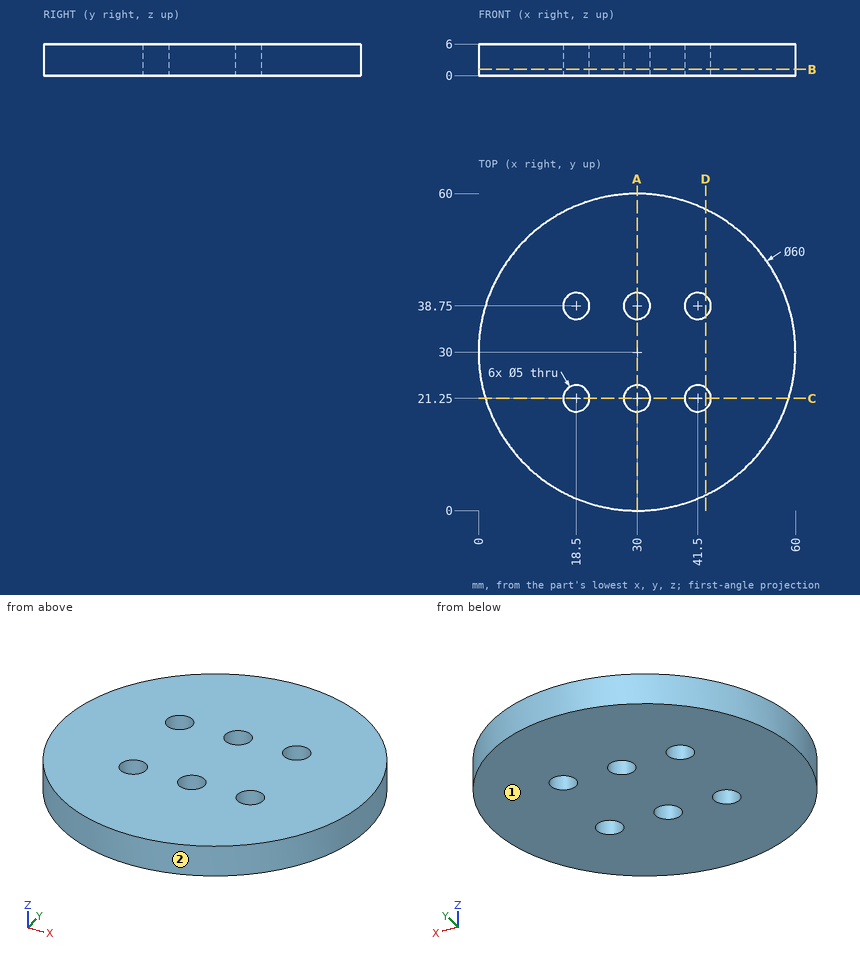
Answer from the drawing. Dimensions are ordinates in mm from the lowest x, y and z of the part. Coordinates: 2 decimals unless noted, no trailing zeros. Loops run counter-clockwise (first coordinate to the right, second up) from the corner with the lowest first, then second, coordinate; pieces in that order, holes last.
Q1. The part is cut by section B-B on z = 1.2. Write down the section's boundary in (x, y).
Q2. The part is cut by section D-D on x = 43. Write down the section's boundary in (y, z).
Q3. The mould has two halves that part along Y. Classify the marked faces 1 and 2: +Y half, -Y half, draft (parallel to the pull), parting line (faces both ways), or undercut.
Q4. The part is cut by section C-C on y = 21.25. Write down the section's boundary in (x, z).
Q5. Each of these flat-tipped pins is pushed along its axis until it touches: pin 1 Ø1 at (y, z) = (23, 4.5) entering from +X; pin 2 Ø3 at (x, z) = (37, 5) entering from -Y. Where does it stop, or does it pass through?
Q6. The part is cut by section A-A on x = 30. Write down the section's boundary in (y, z).
Q7. Consider probe 1 along X at (y, z) = (20.5, 3); probe 2 along Y at (x, z) = (30, 3.4); probe 3 along Y at (x, z) = (41.5, 3). Determine where each line is inside the solid, lowest interval first.
Results below:
1. outline: circle Ø60 at (30, 30); hole circle Ø5 at (18.5, 21.25); hole circle Ø5 at (18.5, 38.75); hole circle Ø5 at (30, 21.25); hole circle Ø5 at (30, 38.75); hole circle Ø5 at (41.5, 21.25); hole circle Ø5 at (41.5, 38.75)
2. outline: (2.96, 0) - (19.25, 0) - (19.25, 6) - (2.96, 6) - close; (23.25, 0) - (36.75, 0) - (36.75, 6) - (23.25, 6) - close; (40.75, 0) - (57.04, 0) - (57.04, 6) - (40.75, 6) - close
3. face 1: draft
3. face 2: parting line
4. outline: (1.3, 0) - (16, 0) - (16, 6) - (1.3, 6) - close; (21, 0) - (27.5, 0) - (27.5, 6) - (21, 6) - close; (32.5, 0) - (39, 0) - (39, 6) - (32.5, 6) - close; (44, 0) - (58.7, 0) - (58.7, 6) - (44, 6) - close
5. pin 1: stops at x = 59.29
5. pin 2: stops at y = 0.51
6. outline: (0, 0) - (18.75, 0) - (18.75, 6) - (0, 6) - close; (23.75, 0) - (36.25, 0) - (36.25, 6) - (23.75, 6) - close; (41.25, 0) - (60, 0) - (60, 6) - (41.25, 6) - close
7. probe 1: x = 1.54 to 16.12, 20.88 to 27.62, 32.38 to 39.12, 43.88 to 58.46
7. probe 2: y = 0 to 18.75, 23.75 to 36.25, 41.25 to 60
7. probe 3: y = 2.29 to 18.75, 23.75 to 36.25, 41.25 to 57.71
